Geometry check sheet. Reference: the model listing, model coordinates, mm. Face numbers are marked on the shaded views. A direction names the side the tool comes from. Coordinates: 2 decimals unless noted, no trailing zeros. Write each loop counter-clockwise with the first axis right and the second up, starting at its lowest first coordinate (ties: lowest second). Pieces come first, ordered by that corner, then holes.
from build123d import *

# Parameters (mm, degrees)
SKETCH2_W           = 25.4
SKETCH2_H           = 25.4
SKETCH2_W_2         = 19.05
SKETCH2_H_2         = 19.05
BOSS_EXTRUDE1_DEPTH = 82.55
CUT_EXTRUDE1_REACH  = 89.298
SKETCH3_W           = 27.94
SKETCH3_H           = 22.225


with BuildPart() as part:
    # Sketch2 → Boss-Extrude1 (new body)
    with BuildSketch(Plane(origin=(0, 0, 0), x_dir=(0, 0, -1), z_dir=(1, 0, 0))):
        Rectangle(SKETCH2_W, SKETCH2_H)
        Rectangle(SKETCH2_W_2, SKETCH2_H_2, mode=Mode.SUBTRACT)
    extrude(amount=BOSS_EXTRUDE1_DEPTH)

    # Cut-Extrude1: up to this face of the body (flat: up to its plane)
    cut_extrude1_end = Plane(part.part.faces().sort_by_distance((41.275, 0, 9.525))[0])
    # Sketch3 → Cut-Extrude1 (cut, up to the picked face)
    with BuildSketch(Plane(origin=(0, 0, -12.7), x_dir=(-1, 0, 0), z_dir=(0, 0, -1)), mode=Mode.PRIVATE) as cut_extrude1_sk1:
        with Locations((-62.23, -1.5875)):
            Rectangle(SKETCH3_W, SKETCH3_H)
    cut_extrude1_tool1 = split(extrude(cut_extrude1_sk1.sketch, amount=-CUT_EXTRUDE1_REACH, mode=Mode.PRIVATE), bisect_by=cut_extrude1_end, keep=Keep.BOTH, mode=Mode.PRIVATE)
    add(cut_extrude1_tool1.solids().sort_by(Axis((62.23, -1.5875, -12.7), (0, 0, 1)))[0], mode=Mode.SUBTRACT)


solid = part.part
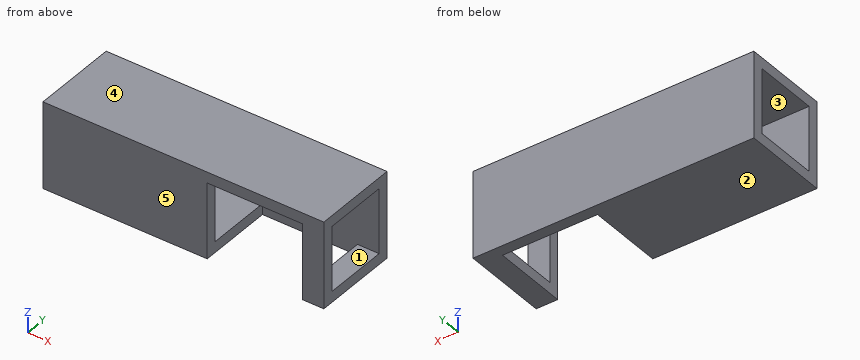
1. Thickness scan on line 1 along Z through (x, y) = (36, -5.75) (3 decimals); line 2 along X through (y, z) = (-10, -1); line 3 along Z through (x, y) = (66, -11.5) (3 decimals). Record the ranges inside material, lowest first.
Computed values:
line 1: z = -12.7 to -9.525, 9.525 to 12.7
line 2: x = 0 to 48.26, 76.2 to 82.55
line 3: z = 9.525 to 12.7
2. Gauge pin test, flat ends, axial feed: pin 1 Ø12 at (y, z) = (-3.5, -8.5) entering from +X; pin 2 Ø11 at (y, z) = (3, -2) entering from +X. Record the tip position at first contact, or that the pin passes through.
Computed values:
pin 1: stops at x = 82.55
pin 2: passes through
3. Sectioned sample at A-A, the plane z = 1.5. Record the boundary of the cut face in (x, y) (3 decimals).
Computed values:
outline: (0, -12.7) - (48.26, -12.7) - (48.26, -9.525) - (0, -9.525) - close; (0, 9.525) - (82.55, 9.525) - (82.55, 12.7) - (0, 12.7) - close; (76.2, -12.7) - (82.55, -12.7) - (82.55, -9.525) - (76.2, -9.525) - close
4. Sectioned sample at D-D, the plane x = 74. Record the boundary of the cut face in (y, z) (3 decimals).
Computed values:
outline: (-12.7, 9.525) - (9.525, 9.525) - (9.525, -12.7) - (12.7, -12.7) - (12.7, 12.7) - (-12.7, 12.7) - close
5. Access from +Z, -Z, +X, -X, +Y, -Y to the whole of each face (thin tool, end or side, straight path). Record for the marked faces 1 and 2.
Computed values:
face 1: +X, -X
face 2: -Z, +X, -X, +Y, -Y
6. Draft check along Z on the marked faces 3, 4 and 5. Enter one of: released by +Z, released by -Z, zero draft, split by the parting line, or undercut.
Computed values:
face 3: undercut
face 4: released by +Z
face 5: zero draft
7. Sectioned sample at C-C, the plane x = 25.5. Record the boundary of the cut face in (y, z) (3 decimals), and give its area (3 significant figures).
Computed values:
outline: (-12.7, -12.7) - (12.7, -12.7) - (12.7, 12.7) - (-12.7, 12.7) - close; hole (-9.525, -9.525) - (9.525, -9.525) - (9.525, 9.525) - (-9.525, 9.525) - close
area: 282 mm2
